```python
from build123d import *

# Parameters (mm, degrees)
SKETCH_1_R          = 5.2
EXTRUDE_1_DEPTH     = 27.5
SKETCH_6_R          = 7.2
EXTRUDE_3_DEPTH     = 1.75
SKETCH_8_R          = 6
EXTRUDE_4_DEPTH     = 23.5
SKETCH_3_R          = 0.85
CUT_EXTRUDE_4_DEPTH = 8
SKETCH_7_R          = 0.9
CUT_EXTRUDE_5_DEPTH = 8
CHAMFER_1_SIZE      = 1
CHAMFER_2_SIZE      = 1
SKETCH_9_R          = 0.493863849
CUT_EXTRUDE_6_DEPTH = 1
CHAMFER_3_SIZE      = 0.8


with BuildPart() as part:
    # 草图1 → 凸台-拉伸1 (new body)
    with BuildSketch(Plane.XY):
        Circle(SKETCH_1_R)
    extrude(amount=EXTRUDE_1_DEPTH)

    # 草图6 → 凸台-拉伸3 (add)
    with BuildSketch(Plane.XY.offset(27.5)):
        Circle(SKETCH_6_R)
    extrude(amount=-EXTRUDE_3_DEPTH)

    # 草图8 → 凸台-拉伸4 (add)
    with BuildSketch(Plane(origin=(0, 0, 25.75), x_dir=(-1, 0, 0), z_dir=(0, 0, -1))):
        with Locations(Location((0, 0, 0), (0, 0, 180))):
            Circle(SKETCH_8_R)
    extrude(amount=EXTRUDE_4_DEPTH)

    # 草图3 → 切除-拉伸4 (cut)
    with BuildSketch(Plane.XY.offset(27.5)):
        with Locations((-3, 0)):
            Circle(SKETCH_3_R)
        with Locations((3, 0)):
            Circle(SKETCH_3_R)
    cut_extrude_4 = extrude(amount=-CUT_EXTRUDE_4_DEPTH, mode=Mode.SUBTRACT)

    # 镜向3: 切除-拉伸4 across plane
    add(cut_extrude_4.mirror(Plane.XY.offset(13.75)), mode=Mode.SUBTRACT)

    # 草图7 → 切除-拉伸5 (cut)
    with BuildSketch(Plane.XY.offset(27.5)):
        with Locations((-3, 0)):
            Circle(SKETCH_7_R)
        with Locations((3, 0)):
            Circle(SKETCH_7_R)
    extrude(amount=-CUT_EXTRUDE_5_DEPTH, mode=Mode.SUBTRACT)

    # 倒角1
    chamfer_1_edges = [part.edges().sort_by_distance(p)[0] for p in [
        (-3.85, 0, 0),
        (2.15, 0, 0),
    ]]
    chamfer(chamfer_1_edges, length=CHAMFER_1_SIZE)

    # 倒角2
    chamfer_2_edges = [part.edges().sort_by_distance(p)[0] for p in [
        (-3.9, 0, 27.5),
        (2.1, 0, 27.5),
    ]]
    chamfer(chamfer_2_edges, length=CHAMFER_2_SIZE)

    # 草图9 → 切除-拉伸6 (cut)
    with BuildSketch(Plane(origin=(0, 0, 0), x_dir=(-1, 0, 0), z_dir=(0, 0, -1))):
        with Locations((-1.600597529, 2.951921672)):
            Circle(SKETCH_9_R)
        with Locations(Location((1.529748789, 2.989251185, 0), (0, 0, 180))):
            Circle(SKETCH_9_R)
        with Locations((1.600597529, -2.951921672)):
            Circle(SKETCH_9_R)
        with Locations(Location((-1.529748789, -2.989251185, 0), (0, 0, 180))):
            Circle(SKETCH_9_R)
    extrude(amount=-CUT_EXTRUDE_6_DEPTH, mode=Mode.SUBTRACT)

    # 倒角3
    chamfer_3_edges = [part.edges().sort_by_distance(p)[0] for p in [
        (-7.2, 0, 27.5),
    ]]
    chamfer(chamfer_3_edges, length=CHAMFER_3_SIZE)


solid = part.part
```
Part model, mm, in its own coordinate system. A direction names the side the tool comes from. Coordinates: 2 decimals unless noted, no trailing zeros. Loops run counter-clockwise (first coordinate to the right, second up) from the corner with the lowest first, then second, coordinate; pieces in that order, holes last. Notation, with made-up numbers: (24.25, 69.25) - (59.25, 69.25) arc R34 ccw to (59.25, 108.25) - close; hole circle Ø9 at (-24, 16). An arc over 180 degrees is marked (long way). Write item = value, one per line. Start each with the question number.
Item 1: Cut at D-D, the plane z = 6.5. Give the cut face in (x, y).
Item 2: Cut at B-B, the plane z = 22. Give the cut face in (x, y), and give its area (3 significant figures).
Item 3: Cut at C-C, the plane z = 18. Give the cut face in (x, y).
Item 4: Flat gauge pins, fed straight in: pin 1 Ø1.9 at (x, y) = (3, -0.5) entering from -Z; pin 2 Ø1 at (x, y) = (3, 1.5) entering from +Z; pin 3 Ø0.8 at (x, y) = (1.5, -3) entering from -Z; pin 4 Ø0.8 at (x, y) = (-3.5, 0.5) entering from -Z. Where does each tip first touch, or does it go through?
Item 5: 3-axis set-ups, long thin cutter, end or side, ignore diameter. For faces 1 (the flat face through (3, 0, 19.5)), 2 (the cylindrical face through (1.986, -2.8, 0.493)): which of +Z, -Z, +X, -X, +Y, -Y reach the whole face in a straight line?
Item 6: Cut at A-A, the plane x = 0. Give the cut face in (y, z).
Item 7: Wall check: L1, parallel to Y at x = -3, z = 21.25; L2, parallel to Y at x = 2.25, z = 24.75; L3, parallel to Z at x = -5.75, y = -1.5. Give the ranges that are in metal, low to high. Write a range as from..to.
Item 8: Mould opens along Y. For faces 3 (the flat face through (0, 0, 0)), 4 (the cylindrical face through (6.87, 2.16, 26.23)), 5 (the cylindrical face through (1.144, 2.763, 0.493)) say: released by +Y, released by -Y, zero draft, split by the parting line, or undercut.
The answers:
q1.outline = circle Ø12 at (0, 0); hole circle Ø1.7 at (-3, 0); hole circle Ø1.7 at (3, 0)
q2.outline = circle Ø12 at (0, 0); hole circle Ø1.8 at (-3, 0); hole circle Ø1.8 at (3, 0)
q2.area = 108 mm2
q3.outline = circle Ø12 at (0, 0)
q4.pin_1 = 0.4
q4.pin_2 = 27.5
q4.pin_3 = 1
q4.pin_4 = 0.74
q5.face_1 = +Z
q5.face_2 = -Z
q6.outline = (-7.2, 25.75) - (-6, 25.75) - (-6, 2.25) - (-5.2, 2.25) - (-5.2, 0) - (5.2, 0) - (5.2, 2.25) - (6, 2.25) - (6, 25.75) - (7.2, 25.75) - (7.2, 26.7) - (6.4, 27.5) - (-6.4, 27.5) - (-7.2, 26.7) - close
q7.L1 = -5.2..-0.9, 0.9..5.2
q7.L2 = -5.56..-0.5, 0.5..5.56
q7.L3 = 2.25..27.5
q8.face_3 = zero draft
q8.face_4 = split by the parting line
q8.face_5 = undercut
